Check sheet for the drawn part. Datum: minimum x, y, z corner. Units: mm. A direction names the side the tool comes from. Give positions to 0.01 mm unless a question says otherwise; leave off trailing zeros. Write each loop counter-clockwise with the first axis right and the second up, starting at its lowest first coordinate (ties: lowest second). Pieces come first, ordered by that corner, then holes. Notation, with made-up numbers: (54.5, -34.75) - (98.5, -34.75) arc R18 cw to (98.5, -13.75) - close; hole circle Ø11 at (-26.5, 57). An arc over 180 degrees is marked (long way). Return JSON: item names as keys, results as strings. Group by question number.
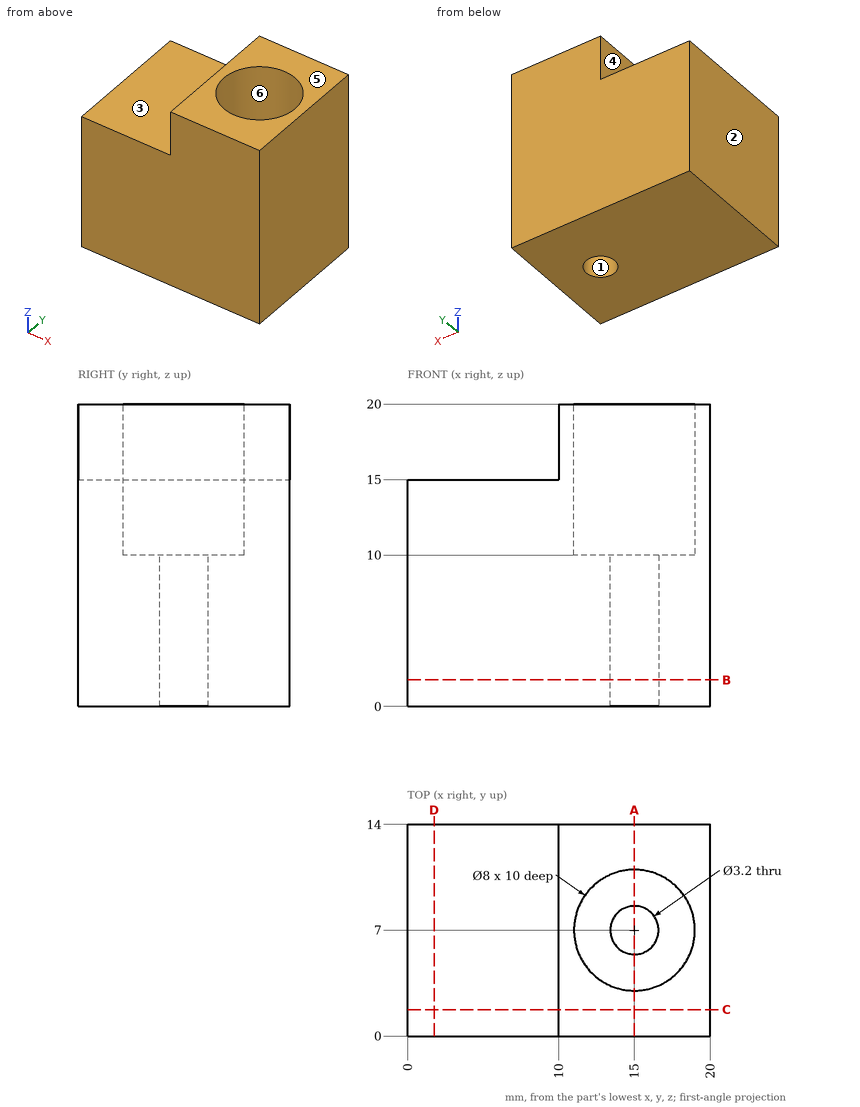
Item 1: Section check A-A on x = 15. Record the cut outline in (y, z).
Item 2: Section check D-D on x = 1.75. Record the cut outline in (y, z), plus the area to 3 significant figures.
Item 3: Section check C-C on y = 1.75. Record the cut outline in (x, z).
Item 4: Depth check by flat-ended pin: pin 1 (5 mm diameter, centred on x = 6.5, y = 8.5, fed in from +Z). Enter the tip coordinate at first touch or a pass-through.
Item 5: Section check B-B on z = 1.75. Record the cut outline in (x, y).
Item 6: Material ranges on line 1 along Y through (x, z) = (15, 5.75); line 2 along Y through (x, z) = (15, 15); line 3 along Z through (x, y) = (6.75, 10.25), recorded low to high. Write a range as from..to.
Item 7: Mould release check, pull along X, two halves, no side actions. Record for the marked faces 1, 2 and 3: +X half, -X half, draft (parallel to the pull), parting line (faces both ways), or undercut.
Item 8: Access from +Z, -Z, +X, -X, +Y, -Y to the whole of each face (thin tool, end or side, straight path). Record for the marked faces 4, 5 and 6.
Reply:
{
 "1": {"outline": "(0, 0) - (5.4, 0) - (5.4, 10) - (3, 10) - (3, 20) - (0, 20) - close; (8.6, 0) - (14, 0) - (14, 20) - (11, 20) - (11, 10) - (8.6, 10) - close"},
 "2": {"outline": "(0, 0) - (14, 0) - (14, 15) - (0, 15) - close", "area": "210 mm²"},
 "3": {"outline": "(0, 0) - (20, 0) - (20, 20) - (10, 20) - (10, 15) - (0, 15) - close"},
 "4": {"pin 1": "z = 15"},
 "5": {"outline": "(0, 0) - (20, 0) - (20, 14) - (0, 14) - close; hole circle Ø3.2 at (15, 7)"},
 "6": {"line 1": "0..5.4, 8.6..14", "line 2": "0..3, 11..14", "line 3": "0..15"},
 "7": {"face 1": "undercut", "face 2": "-X half", "face 3": "draft"},
 "8": {"face 4": "+Z, -X, +Y, -Y", "face 5": "+Z, +X, -X, +Y, -Y", "face 6": "+Z"}
}
